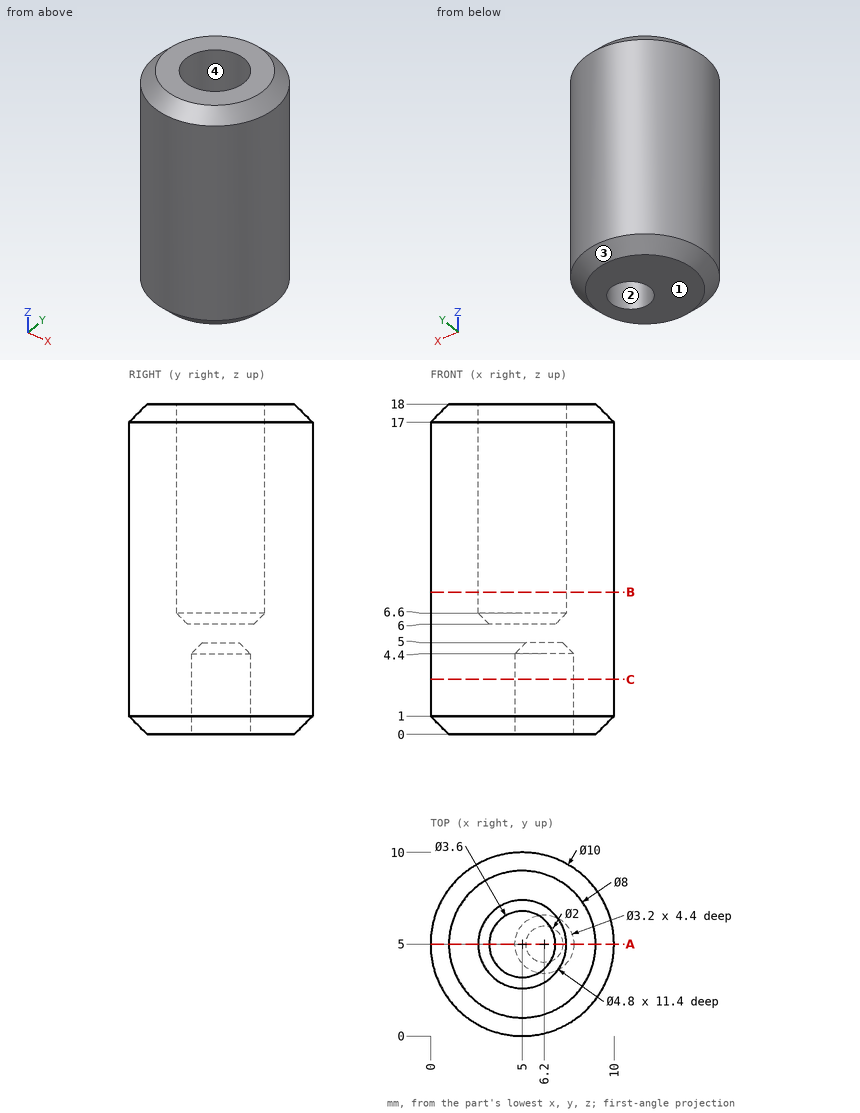
Study the drawing (mm; zero at the part's minimum x, y, z) and answer. Give positions to 0.01 mm unless a question says otherwise; leave off trailing zeros. Write each loop counter-clockwise with the first axis right and the second up, starting at its lowest first coordinate (ties: lowest second). Pieces come first, ordered by that corner, then holes. Notation, with made-up numbers: (9.25, -17) -> (23.25, -17) arc R12 cw to (23.25, -5) -> close; hole circle Ø8 at (-6, 56). An arc over 180 degrees is marked (long way). Answer as a JSON object with one key per item and string values. Group by question number.
1) The mould has two halves that part along X. Classify the marked faces 1, 2, 3 and 4: +X half, -X half, draft (parallel to the pull), parting line (faces both ways), or undercut.
2) Find section B-B (z = 7.75). Write down the section's boundary in (x, y).
3) Find section A-A (y = 5). Write down the section's boundary in (x, z).
4) Consider L1, parallel to Y at x = 5, z = 9.25; L2, parallel to X at y = 5.75, z = 14.5; L3, parallel to Z at x = 6, y = 5.75. Determine where each line is inside the solid, lowest interval first. Write a range as from..to.
5) Each of these flat-tipped pins is pushed along its axis until it touches: P1, Ø1, axis at y = 6.5, z = 13, coming from the -X side; P2, Ø1, axis at x = 4, z = 15, coming from the -Y side; P3, Ø1, axis at x = 6.5, y = 4.5, coming from the -Z side. Where does it stop, or does it pass through?
6) Find section C-C (z = 3). Write down the section's boundary in (x, y).
Values follow:
{
 "1": {"face 1": "draft", "face 2": "undercut", "face 3": "parting line", "face 4": "undercut"},
 "2": {"outline": "circle Ø10 at (5, 5); hole circle Ø4.8 at (5, 5)"},
 "3": {"outline": "(0, 1) -> (1, 0) -> (4.6, 0) -> (4.6, 4.4) -> (5.2, 5) -> (7.2, 5) -> (7.8, 4.4) -> (7.8, 0) -> (9, 0) -> (10, 1) -> (10, 17) -> (9, 18) -> (7.4, 18) -> (7.4, 6.6) -> (6.8, 6) -> (3.2, 6) -> (2.6, 6.6) -> (2.6, 18) -> (1, 18) -> (0, 17) -> close"},
 "4": {"L1": "y = 0..2.6, 7.4..10", "L2": "x = 0.06..2.72, 7.28..9.94", "L3": "z = 5..6"},
 "5": {"P1": "stops at x = 0.1", "P2": "stops at y = 0.03", "P3": "stops at z = 4.92"},
 "6": {"outline": "circle Ø10 at (5, 5); hole circle Ø3.2 at (6.2, 5)"}
}
